Input: part model. Units: mm. Frame: model coordinates. Face numbers are marked on the shaded views. Coordinates: 2 decimals unless noted, no trailing zeros. Order: outer loops, then holes, each group sorted by start corner. A loop starts at its lowest first (then second) coordinate and runs counter-clockwise, first axis right, second up. Notation, with made-up numbers: M -6,88.5 L 31,88.5 A32 cw 31,117.5 Z; hole C -19,74 d11. An arc over 180 degrees is marked long. One line per item, written item: value.
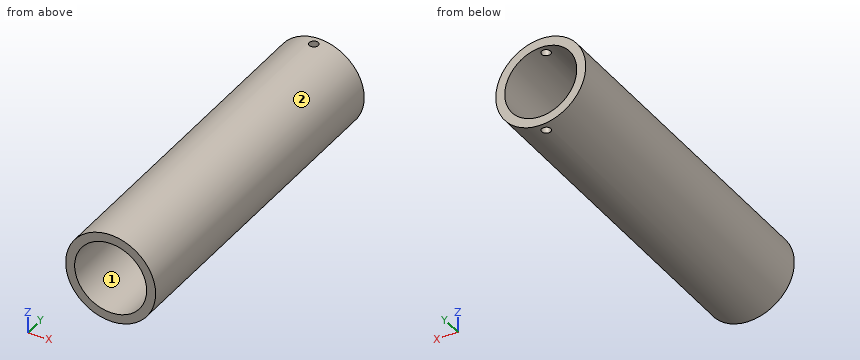
```python
from build123d import *

# Parameters (mm, degrees)
SKETCH001_R  = 2.5
PAD001_DEPTH = 30
SKETCH_R     = 25
SKETCH_R_2   = 20
PAD_DEPTH    = 95


with BuildPart() as pad001:
    # Sketch001 → Pad001 (new body, symmetric)
    with BuildSketch(Plane.XY):
        with Locations((0, 90)):
            Circle(SKETCH001_R)
    extrude(amount=PAD001_DEPTH, both=True)


with BuildPart() as cut:
    # Sketch → Pad (new body, symmetric)
    with BuildSketch(Plane.XZ):
        Circle(SKETCH_R)
        Circle(SKETCH_R_2, mode=Mode.SUBTRACT)
    extrude(amount=PAD_DEPTH, both=True)

    # Cut: cut Pad001
    add(pad001.part, mode=Mode.SUBTRACT)


solid = cut.part
```
(1) Draft query along X for the marked faces 1 and 2. Return one class per face: released by +X, released by -X, zero draft, split by the parting line, or undercut.
Data:
face 1: undercut
face 2: split by the parting line
(2) First-contact query: pin 1 (6 mm diameter, centred on x = 1, y = -46, fed in from -Z); pin 2 (4 mm diameter, centred on x = -14, y = -20, fed in from -Z); pin 3 (1.5 mm diameter, centred on x = -10.5, y = -30.5, fed in from +Z). Flat tips, straight axial feed; report the tip coordinate or a pass-through.
Data:
pin 1: stops at z = -25
pin 2: stops at z = -21.93
pin 3: stops at z = 23.02
(3) Cut plane B-B on z = 0. Output: boundary loops of the cut face in (x, y).
Data:
outline: M -25,-95 L -20,-95 L -20,95 L -25,95 Z; M 20,-95 L 25,-95 L 25,95 L 20,95 Z
(4) Ray query, line 1 (Z direction, x = 0, y = 9); line 2 (Y direction, x = 0, z = 22); line 3 (X direction, y = 90, z = -20.85). Return the intervals inside material, ascending. Write a range as from..to.
Data:
line 1: z = -25..-20, 20..25
line 2: y = -95..87.5, 92.5..95
line 3: x = -13.79..-2.5, 2.5..13.79
(5) Cut plane D-D on y = 90. Output: boundary loops of the cut face in (x, z), plus the area to 3 significant figures.
Data:
outline: M -2.5,-24.87 L -2.5,-19.84 A20 cw -2.5,19.84 L -2.5,24.87 A25 ccw Z; M 2.5,-24.87 A25 ccw 2.5,24.87 L 2.5,19.84 A20 cw 2.5,-19.84 Z
area: 657 mm2
(6) Cut plane A-A on x = 0. Output: boundary loops of the cut face in (y, z).
Data:
outline: M -95,-25 L 87.5,-25 L 87.5,-20 L -95,-20 Z; M -95,20 L 87.5,20 L 87.5,25 L -95,25 Z; M 92.5,-25 L 95,-25 L 95,-20 L 92.5,-20 Z; M 92.5,20 L 95,20 L 95,25 L 92.5,25 Z
(7) Cut plane C-C on y = -47. Output: boundary loops of the cut face in (x, z).
Data:
outline: C 0,0 d50; hole C 0,0 d40
